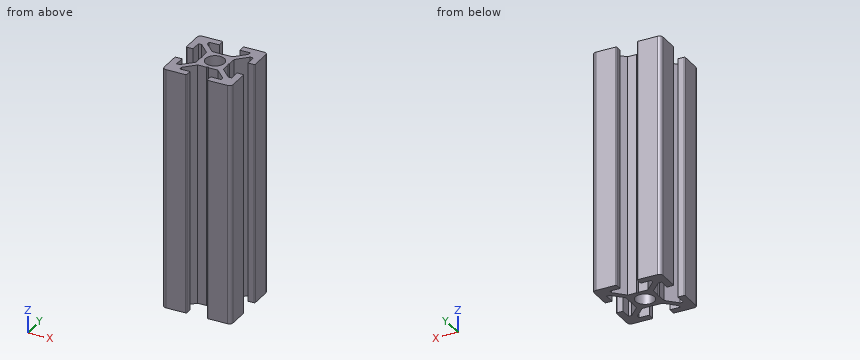
Autodesk Inventor part; units mm, degrees
ref_plane "Startebene" through (0, 0, 0) normal (0, 0, 1) x (1, 0, 0)
ref_plane "Endebene" through (0, 0, 320) normal (0, 0, 1) x (1, 0, 0)
ref_plane "Startebene1" through (0, 0, 0) normal (0, 0, 1) x (1, 0, 0)
ref_plane "Startebene" through (0, 0, 0) normal (0, 0, 1) x (1, 0, 0)
ref_plane "Endebene" through (0, 0, 320) normal (0, 0, 1) x (1, 0, 0)
ref_plane "Startebene1" through (0, 0, 0) normal (0, 0, 1) x (1, 0, 0)
ref_plane "Endebene1" through (0, 0, 40) normal (0, 0, 1) x (1, 0, 0)
ref_plane "Startebene2" through (0, 0, 0) normal (0, 0, 1) x (1, 0, 0)
ref_plane "Endebene2" through (0, 0, 40) normal (0, 0, 1) x (1, 0, 0)
ref_plane "Startebene3" through (0, 0, 0) normal (0, 0, 1) x (1, 0, 0)
ref_plane "Endebene3" through (0, 0, 70) normal (0, 0, 1) x (1, 0, 0)
sketch "Skizze" plane through (0, 0, 0) normal (0, 0, 1) x (1, 0, 0)
  line L0 (-10, 9) -> (-10, 3.3)
  arc A0 (-10, 3.3) -> (-9.7, 3) centre (-9.7, 3.3) ccw
  line L1 (-9.7, 3) -> (-8, 3)
  line L2 (-8, 3) -> (-8, 6)
  line L3 (-8, 6) -> (-7.0607, 6)
  line L4 (-7.0607, 6) -> (-4, 2.9393)
  line L5 (-4, 2.9393) -> (-4, 0.3)
  line L6 (-4, 0.3) -> (-3.7, 0)
  line L7 (-3.7, 0) -> (-4, -0.3)
  line L8 (-4, -0.3) -> (-4, -2.9393)
  line L9 (-4, -2.9393) -> (-7.0607, -6)
  line L10 (-7.0607, -6) -> (-8, -6)
  line L11 (-8, -6) -> (-8, -3)
  line L12 (-8, -3) -> (-9.7, -3)
  arc A1 (-9.7, -3) -> (-10, -3.3) centre (-9.7, -3.3) ccw
  line L13 (-10, -3.3) -> (-10, -9)
  arc A2 (-10, -9) -> (-9, -10) centre (-9, -9) ccw
  line L14 (-9, -10) -> (-3.3, -10)
  arc A3 (-3.3, -10) -> (-3, -9.7) centre (-3.3, -9.7) ccw
  line L15 (-3, -9.7) -> (-3, -8)
  line L16 (-3, -8) -> (-6, -8)
  line L17 (-6, -8) -> (-6, -7.0607)
  line L18 (-6, -7.0607) -> (-2.9393, -4)
  line L19 (-2.9393, -4) -> (-0.3, -4)
  line L20 (-0.3, -4) -> (0, -3.7)
  line L21 (0, -3.7) -> (0.3, -4)
  line L22 (0.3, -4) -> (2.9393, -4)
  line L23 (2.9393, -4) -> (6, -7.0607)
  line L24 (6, -7.0607) -> (6, -8)
  line L25 (6, -8) -> (3, -8)
  line L26 (3, -8) -> (3, -9.7)
  arc A4 (3, -9.7) -> (3.3, -10) centre (3.3, -9.7) ccw
  line L27 (3.3, -10) -> (9, -10)
  arc A5 (9, -10) -> (10, -9) centre (9, -9) ccw
  line L28 (10, -9) -> (10, -3.3)
  arc A6 (10, -3.3) -> (9.7, -3) centre (9.7, -3.3) ccw
  line L29 (9.7, -3) -> (8, -3)
  line L30 (8, -3) -> (8, -6)
  line L31 (8, -6) -> (7.0607, -6)
  line L32 (7.0607, -6) -> (4, -2.9393)
  line L33 (4, -2.9393) -> (4, -0.3)
  line L34 (4, -0.3) -> (3.7, 0)
  line L35 (3.7, 0) -> (4, 0.3)
  line L36 (4, 0.3) -> (4, 2.9393)
  line L37 (4, 2.9393) -> (7.0607, 6)
  line L38 (7.0607, 6) -> (8, 6)
  line L39 (8, 6) -> (8, 3)
  line L40 (8, 3) -> (9.7, 3)
  arc A7 (9.7, 3) -> (10, 3.3) centre (9.7, 3.3) ccw
  line L41 (10, 3.3) -> (10, 9)
  arc A8 (10, 9) -> (9, 10) centre (9, 9) ccw
  line L42 (9, 10) -> (3.3, 10)
  arc A9 (3.3, 10) -> (3, 9.7) centre (3.3, 9.7) ccw
  line L43 (3, 9.7) -> (3, 8)
  line L44 (3, 8) -> (6, 8)
  line L45 (6, 8) -> (6, 7.0607)
  line L46 (6, 7.0607) -> (2.9393, 4)
  line L47 (2.9393, 4) -> (0.3, 4)
  line L48 (0.3, 4) -> (0, 3.7)
  line L49 (0, 3.7) -> (-0.3, 4)
  line L50 (-0.3, 4) -> (-2.9393, 4)
  line L51 (-2.9393, 4) -> (-6, 7.0607)
  line L52 (-6, 7.0607) -> (-6, 8)
  line L53 (-6, 8) -> (-3, 8)
  line L54 (-3, 8) -> (-3, 9.7)
  arc A10 (-3, 9.7) -> (-3.3, 10) centre (-3.3, 9.7) ccw
  line L55 (-3.3, 10) -> (-9, 10)
  arc A11 (-9, 10) -> (-10, 9) centre (-9, 9) ccw
  circle A12 centre (0, 0) radius 2.75
  dimension "d2" = 5.5
  dimension "d3" = 10
  dimension "d4" = 10
  dimension "d5" = 5.7
  dimension "d6" = 5.7
  dimension "d7" = 1.7
  dimension "d8" = 3
  dimension "d9" = 0.3
  dimension "d10" = 90
  dimension "d11" = 45
  dimension "d12" = 45
  dimension "d13" = 45
  dimension "d14" = 90
  dimension "d15" = 90
  dimension "d16" = 45
  dimension "d17" = 45
  dimension "d18" = 45
  dimension "d19" = 45
  dimension "d20" = 90
  dimension "d21" = 90
  dimension "d22" = 45
  dimension "d23" = 45
  dimension "d24" = 90
  dimension "d25" = 90
  dimension "d26" = 90
  dimension "d27" = 90
  dimension "d28" = 90
  dimension "d29" = 90
  dimension "d30" = 90
  dimension "d31" = 90
  dimension "d32" = 90
  dimension "d33" = 90
  dimension "d34" = 90
  dimension "d35" = 90
  dimension "d36" = 90
  dimension "d37" = 90
  dimension "d38" = 90
  dimension "d39" = 4
  dimension "d40" = 6
  dimension "d41" = 13
  dimension "d42" = 14
  dimension "d43" = 16
  dimension "d44" = 18
  dimension "d45" = 3
  dimension "d46" = 9
  dimension "d47" = 7
  dimension "d48" = 1
  dimension "d49" = 7
  dimension "d50" = 1.5
  dimension "d51" = 1.8663
  dimension "d52" = 3.3663
  dimension "d53" = 1.5
  dimension "d54" = 1.8663
  dimension "d55" = 3.3663
  dimension "d56" = 4
  dimension "d57" = 10.8187
  dimension "d58" = 1.9092
  dimension "d59" = 5
  dimension "d60" = 13
  dimension "d61" = 13
  dimension "d62" = 16.0513
  dimension "d63" = 3.3234
  dimension "d64" = 14
  dimension "d65" = 12.685
extrude "Körper" add sketch "Skizze" along normal up to surface (70 mm away) from surface at 0
sketch "Skizze21" plane through (0, 0, 0) normal (0, 0, 1) x (1, 0, 0)
  line L0 (0, 0) -> (10, 0)
ref_plane "Arbeitsebene18" through (0, 0, 0) normal (0, -1, 0) x (1, 0, 0)
sketch "Skizze22" plane through (0, 0, 0) normal (0, -1, 0) x (1, 0, 0)
  line L0 (-2, 0) -> (12, 0)
  line L1 (-2, 70) -> (12, 70)
  dimension "d80" = 70
equation "\"G_OFFSET_START\" = 0"
equation "\"G_OFFSET_END\" = 0"
equation "\"G_L\" = d80"
equation "\"G_OFFSET_START1\" = 0"
equation "\"G_OFFSET_END1\" = 0"
equation "\"G_OFFSET_START2\" = 0"
equation "\"G_OFFSET_END2\" = 0"
equation "\"G_OFFSET_START3\" = 0"
equation "\"G_OFFSET_END3\" = 0"
properties part number "Alu Profil 20x20 - AP2020"
Read the model definition and answer for the solid it produces. Units are mm, in the model's axes. Coordinates: 2 decimals unless noted, no trailing zeros. Loops run counter-clockwise (first coordinate to the right, second up) from the corner with the lowest first, then second, coordinate; pieces in that order, holes last. Notation, with made-up numbers: (22.5, -8) - (62.5, -8) arc R14 ccw to (62.5, 5) - close; hole circle Ø11 at (33.5, 88.5). An arc over 180 degrees is marked (long way). Answer in a Markdown table with one row per item.
Q1. Given P1, Ø4, axis at y = 2.5, z = 36.5, coming from the -X side; P2, Ø2, axis at x = -1.5, z = 37.5, coming from the -Y side; P3, Ø2, axis at y = 1, z = 20.5, coming from the +X side; P4, Ø1.5, axis at x = -1.5, z = 34, coming from the +Y side, each flat-ended and moving along its own axis, determine where each tip first touches the part or whether it passes through.
Here are the results:
| item | result |
|---|---|
| P1 | stops at x = -10 |
| P2 | stops at y = -4 |
| P3 | stops at x = 4 |
| P4 | stops at y = 4 |
Q2. Straight lines are drawn through the part: line 1 along Y through (x, z) = (-5, 40); line 2 along Y through (x, z) = (-3.5, 48); line 3 along Y through (x, z) = (-4.5, 16). For each, find the intervals that lie inside material, in ascending order. Write a range as [from, to].
Here are the results:
| item | result |
|---|---|
| line 1 | y = [-10, -8], [-6.06, -3.94], [3.94, 6.06], [8, 10] |
| line 2 | y = [-10, -8], [-4.56, 4.56], [8, 10] |
| line 3 | y = [-10, -8], [-5.56, -3.44], [3.44, 5.56], [8, 10] |
Q3. Find section B-B on y = 2. Write down the section's boundary in (x, z), plus the area to 3 significant figures.
Here are the results:
| item | result |
|---|---|
| outline | (-4, 0) - (-1.89, 0) - (-1.89, 70) - (-4, 70) - close; (1.89, 0) - (4, 0) - (4, 70) - (1.89, 70) - close |
| area | 296 mm^2 |
Q4. Find section A-A on y = 5. Write down the section's boundary in (x, z).
Here are the results:
| item | result |
|---|---|
| outline | (-10, 0) - (-8, 0) - (-8, 70) - (-10, 70) - close; (-6.06, 0) - (-3.94, 0) - (-3.94, 70) - (-6.06, 70) - close; (3.94, 0) - (6.06, 0) - (6.06, 70) - (3.94, 70) - close; (8, 0) - (10, 0) - (10, 70) - (8, 70) - close |
